The listing builds one solid part. Answer for the finished solid, in the listing's coordinates (mm). A direction names the side the tool comes from. Give positions to 0.01 mm unless a question says otherwise; leave off trailing zeros. Order: outer loops, then holes, each group sorted by start corner. A loop starts at its lowest first (then second) coordinate and runs counter-clockwise, first axis right, second up. Notation, with made-up numbers: (58.25, 46) - (92.25, 46) arc R22 ccw to (92.25, 69) - close; hole circle Ø8 at (16, 61.5). An arc over 180 degrees is marked (long way). Use CSV: the item, a comma, the result in double quotes.
```python
from build123d import *

# Parameters (mm, degrees)
SKETCH1_W           = 86
SKETCH1_H           = 141.3
BOSS_EXTRUDE1_DEPTH = 4
SKETCH1_3_W         = 86
SKETCH1_3_H         = 141.3
SKETCH1_3_W_2       = 74
SKETCH1_3_H_2       = 129.3
BOSS_EXTRUDE2_DEPTH = 6
BOSS_EXTRUDE3_DEPTH = 10
FILLET2_R           = 2.5


with BuildPart() as part:
    # Sketch1 → Boss-Extrude1 (new body)
    with BuildSketch(Plane(origin=(0, 0, 0), x_dir=(1, 0, 0), z_dir=(0, 1, 0))):
        Rectangle(SKETCH1_W, SKETCH1_H)
    extrude(amount=BOSS_EXTRUDE1_DEPTH)

    # Sketch1<3> → Boss-Extrude2 (add)
    with BuildSketch(Plane(origin=(0, 0, 0), x_dir=(1, 0, 0), z_dir=(0, 1, 0))):
        Rectangle(SKETCH1_3_W, SKETCH1_3_H)
        Rectangle(SKETCH1_3_W_2, SKETCH1_3_H_2, mode=Mode.SUBTRACT)
    extrude(amount=-BOSS_EXTRUDE2_DEPTH)

    # Sketch2 → Boss-Extrude3 (add)
    with BuildSketch(Plane(origin=(0, 4, 0), x_dir=(1, 0, 0), z_dir=(0, 1, 0))):
        Polygon((-43, 49.188592066), (-53, 22.225), (-53, -22.225), (-43, -49.188592066), (-43, -22.225), (-43, -14.605), (-48, -14.605), (-48, 14.605), (-43, 14.605), (-43, 22.225), align=None)
        Polygon((53, 22.225), (43, 22.225), (43, 14.605), (48, 14.605), (48, -14.605), (43, -14.605), (43, -22.225), (43, -49.188592066), (53, -22.225), align=None)
        Polygon((43, 49.188592066), (43, 22.225), (53, 22.225), align=None)
    extrude(amount=-BOSS_EXTRUDE3_DEPTH)

    # Fillet2
    fillet2_edges = [part.edges().sort_by_distance(p)[0] for p in [
        (0, 4, 70.65),
        (43, 4, -59.919296033),
        (-43, 4, 59.919296033),
        (0, 4, -70.65),
        (-48, 4, -35.706796033),
        (-53, -1, -22.225),
        (-43, -1, -49.188592066),
        (-43, -1, 49.188592066),
        (-53, 4, 0),
        (-48, 4, 35.706796033),
        (-48, 4, 0),
        (43, 4, 59.919296033),
        (43, -1, -49.188592066),
        (53, 4, 0),
        (53, -1, -22.225),
        (48, 4, 35.706796033),
        (53, -1, 22.225),
        (43, -1, 49.188592066),
        (48, 4, 0),
        (-43, 4, -59.919296033),
        (48, 4, -35.706796033),
        (43, -1, -70.65),
        (43, -1, 70.65),
        (-43, -1, 70.65),
        (-43, -1, -70.65),
    ]]
    fillet(fillet2_edges, radius=FILLET2_R - 0.0001)  # a hair under: the kernel refuses the full size


solid = part.part
```
Item 1: The part is cut by section C-C (y = -2.75). Count the separate pieces of the cut face and the enclosed holes in it, and give its area (3 significant figures).
Taken from the geometry:
separate pieces,"1"
enclosed holes,"3"
area,"3,710 mm^2"
Item 2: Which of the six approach directions +Z, -Z, +X, -X, +Y, -Y give full straight-line access (tool end or side, diameter ignored) to faces 1 (the face through (43, -1, 0)), 2 (the face through (-37, -3, 1)), 3 (the face through (-43, -2, -59)), 4 (the face through (-43, -2, 59)), 5 (the face through (43, -2, 59))?
Taken from the geometry:
face 1,"+Y, -Y"
face 2,"-Y"
face 3,"-Z, -X, +Y, -Y"
face 4,"+Z, -X, +Y, -Y"
face 5,"+Z, +X, +Y, -Y"
Item 3: The part is cut by section A-A (x = 6). Give the vertices of the cut face in (y, z).
Taken from the geometry:
outline,"(-6, -70.65) - (1.5, -70.65) arc R2.5 ccw to (4, -68.15) - (4, 68.15) arc R2.5 ccw to (1.5, 70.65) - (-6, 70.65) - (-6, 64.65) - (0, 64.65) - (0, -64.65) - (-6, -64.65) - close"
Item 4: The mould has two halves that part along X. Classify faces 6 (the face through (48, -2, 0)), 7 (the face through (-1, 4, -1)), 8 (the face through (-53, -2, 0)): +X half, -X half, draft (parallel to the pull), parting line (faces both ways), or undercut.
Taken from the geometry:
face 6,"undercut"
face 7,"draft"
face 8,"-X half"
Item 5: Find the intervals of material crossed by line 1 along X through (y, z) = (-4.5, 0.5); line 2 along Z through (x, y) = (36.5, -2.5); line 3 along X through (y, z) = (-3, -59), in increasing order.
Taken from the geometry:
line 1,"-53 to -48, -43 to -37, 37 to 43, 48 to 53"
line 2,"-70.65 to -64.65, 64.65 to 70.65"
line 3,"-43 to -37, 37 to 43"
Item 6: Each of these flat-tipped pins is pushed along its axis until it touches: pin 1 (10 mm diameter, centred on x = 1, z = -16.5, fed in from -Y); pin 2 (5 mm diameter, centred on y = -2, z = -28, fed in from +X); pin 3 (1.5 mm diameter, centred on y = 1.5, z = -39.5, fed in from -X). Where does it stop, or does it pass through?
Taken from the geometry:
pin 1,"y = 0"
pin 2,"x = 51.79"
pin 3,"x = -46.87"
Item 7: The part is cut by section B-B (z = -53). Give the vertices of the cut face in (x, y).
Taken from the geometry:
outline,"(-43, -6) - (-37, -6) - (-37, 0) - (37, 0) - (37, -6) - (43, -6) - (43, 1.5) arc R2.5 ccw to (40.5, 4) - (-40.5, 4) arc R2.5 ccw to (-43, 1.5) - close"
